Geometry check sheet. Reference: drawing and pictorial views, mm from the part's lowest x, y, z. A direction names the side the tool comes from. Coordinates: 2 decimals unless noted, no trailing zeros. Write each loop counter-clockwise with the first axis right and the second up, starting at its lowest first coordinate (ties: lowest second). Pieces come first, ordered by that corner, then holes. Notation, with made-up numbers: (61, -28.5) -> (77, -28.5) arc R30 cw to (77, 5.5) -> close; hole circle Ø6 at (-3.75, 43). An arc over 180 degrees is marked (long way). Use a Markdown table: item, result. Add a question column.
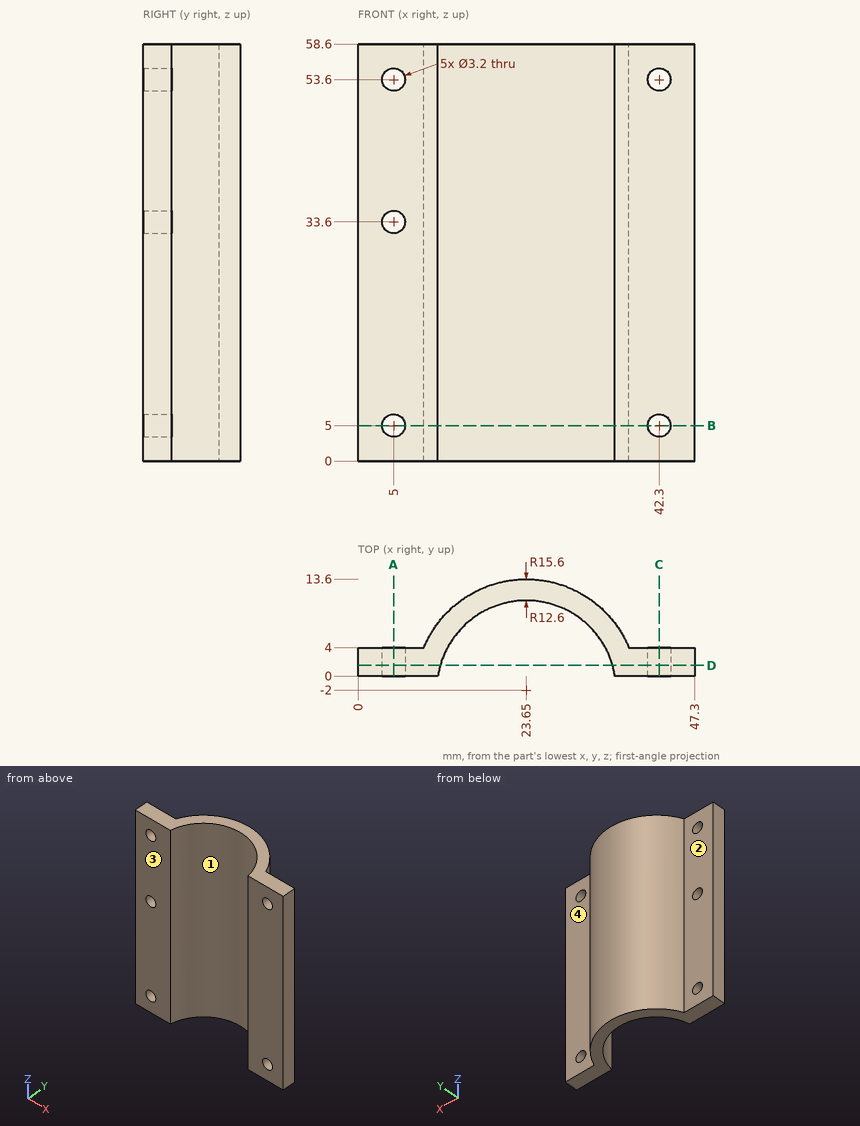
1) Cross-section at B-B on z = 5. Record the boundary of the cut face in (x, y), then the cut area to 3 significant figures.
2) Gauge pin test, flat ends, axial feed: pin 1 (10 mm diameter, centred on x = 3.5, z = 21, fed in from +Y); pin 2 (4 mm diameter, centred on x = 32, z = 21, fed in from +Y); pin 3 (7.5 mm diameter, centred on x = 40.5, z = 41, fed in from +Y). Record the tip position at first contact, or that the pin passes through.
3) Cross-section at A-A on x = 5. Record the boundary of the cut face in (y, z).
4) Cross-section at C-C on x = 42.3. Record the boundary of the cut face in (y, z), then the cut area to 3 significant figures.
5) Release check for a two-part mould opening along Y. For the marked faces 1 and 2 record: released by +Y, released by -Y, zero draft, split by the parting line, or undercut.
6) Thickness scan on L1, parallel to Z at x = 42.3, y = 1; L2, parallel to Z at x = 5, y = 2.7; L3, parallel to X at y = 2.9, z = 5. Record the ranges inside material, lowest first.
7) Set-up check for the marked faces 3 and 4: record each of +Z, -Z, +X, -X, +Y, -Y from which the full face is reachable in a straight line by a thin tool's end or side.
8) Cross-section at D-D on y = 1.5. Record the boundary of the cut face in (x, z), then the cut area to 3 significant figures.
Returned:
| question | item | result |
|---|---|---|
| 1 | outline | (0, 0) -> (3.4, 0) -> (3.4, 4) -> (0, 4) -> close; (6.6, 0) -> (11.21, 0) arc R12.6 cw to (36.09, 0) -> (40.7, 0) -> (40.7, 4) -> (38.05, 4) arc R15.6 ccw to (9.25, 4) -> (6.6, 4) -> close; (43.9, 0) -> (47.3, 0) -> (47.3, 4) -> (43.9, 4) -> close |
| 1 | area | 164 mm² |
| 2 | pin 1 | stops at y = 4 |
| 2 | pin 2 | stops at y = 12.25 |
| 2 | pin 3 | stops at y = 6.47 |
| 3 | outline | (0, 0) -> (4, 0) -> (4, 3.4) -> (0, 3.4) -> close; (0, 6.6) -> (4, 6.6) -> (4, 32) -> (0, 32) -> close; (0, 35.2) -> (4, 35.2) -> (4, 52) -> (0, 52) -> close; (0, 55.2) -> (4, 55.2) -> (4, 58.6) -> (0, 58.6) -> close |
| 4 | outline | (0, 0) -> (4, 0) -> (4, 3.4) -> (0, 3.4) -> close; (0, 6.6) -> (4, 6.6) -> (4, 52) -> (0, 52) -> close; (0, 55.2) -> (4, 55.2) -> (4, 58.6) -> (0, 58.6) -> close |
| 4 | area | 209 mm² |
| 5 | face 1 | released by -Y |
| 5 | face 2 | released by +Y |
| 6 | L1 | z = 0 to 3.4, 6.6 to 52, 55.2 to 58.6 |
| 6 | L2 | z = 0 to 3.4, 6.6 to 32, 35.2 to 52, 55.2 to 58.6 |
| 6 | L3 | x = 0 to 3.4, 6.6 to 12.04, 35.26 to 40.7, 43.9 to 47.3 |
| 7 | face 3 | +Z, -Z, +X, -X, -Y |
| 7 | face 4 | +Z, -Z, +X, +Y |
| 8 | outline | (0, 0) -> (11.55, 0) -> (11.55, 58.6) -> (0, 58.6) -> close; (35.75, 0) -> (47.3, 0) -> (47.3, 58.6) -> (35.75, 58.6) -> close; hole circle Ø3.2 at (5, 5); hole circle Ø3.2 at (5, 33.6); hole circle Ø3.2 at (5, 53.6); hole circle Ø3.2 at (42.3, 5); hole circle Ø3.2 at (42.3, 53.6) |
| 8 | area | 1,310 mm² |
